Geometry check sheet. Reference: the model listing, model coordinates, mm. A direction names the side the tool comes from. Round coordinates to 2 decimals unless told otherwise and drop trailing zeros. Write each loop counter-clockwise with the first axis right and the second up, starting at its lowest first coordinate (ties: lowest second). Pieces come first, ordered by that corner, then holes.
Item 1: Cross-section at A-A (z = 1.75). State how many separate pieces and enclosed holes the cut face has, then the cut area to 3 significant figures.
Item 2: Cross-section at B-B (y = -4.5). Enter the section's corners in (x, z).
Item 3: Draft check along X on faces 1 (the face through (5.3, 0, 1)), 2 (the face through (0, -1.25, -1)), 3 (the face through (-10, 0, 4)). Enter one of: pulls with the +X half, pulls with the -X half, needs draft (parallel to the pull), parting line crosses it, or undercut.
Item 4: Depth check by flat-ended pin: P1, Ø0.6, axis at x = 5.5, z = 2, coming from the +Y side; P2, Ø0.6, axis at x = 0.5, z = -1.5, coming from the -Y side; P3, Ø0.6, axis at y = -2, z = 1.5, coming from the -X side. Enter the tip coordinate at first touch or a pass-through.
Item 5: Scan lines: probe 1 along Z at (x, y) = (-3.5, 2.25); probe 2 along X at (y, z) = (-2, 2.5); probe 3 along X at (y, z) = (-1.75, 1.5). Record each from-to range of solid material in increasing order.
Item 6: Cross-section at C-C (x = 9). Enter the section's corners in (y, z).
Item 7: Access from +Z, -Z, +X, -X, +Y, -Y to the whole of each face (thin tool, end or side, straight path). Record for faces 4 (the face through (0, 1.25, -1)), 5 (the face through (0, -2, 0)), 6 (the face through (-0.1, -2.1, 2.6)), 7 (the face through (0, -6.5, 4)), 8 (the face through (-5.3, 0, 1)).
from build123d import *

# Parameters (mm, degrees)
F1_DEPTH = 2.6
F2_W     = 10.6
F2_H     = 2.5
F3_DEPTH = 2
F5_DEPTH = 0.6
F7_DEPTH = 2
F9_DEPTH = 2
F9_TAPER = 7


# Not quite as in the source:
# - a feature names something its author has since deleted; it is built from what else it names


with BuildPart() as f1:
    # F0 (on Top) → F1 (new body)
    with BuildSketch(Plane.XY):
        Polygon((6, 2.5), (-6, 2.5), (-6, 1.25), (-5.3, 1.25), (-5.3, -1.25), (-6, -1.25), (-6, -2.5), (6, -2.5), (6, -1.25), (5.3, -1.25), (5.3, 1.25), (6, 1.25), align=None)
    extrude(amount=F1_DEPTH)

    # F2 (on face) → F3 (join)
    with BuildSketch(Plane(origin=(0, 0, 0), x_dir=(1, 0, 0), z_dir=(0, 0, -1))):
        Rectangle(F2_W, F2_H)
    extrude(amount=F3_DEPTH)

    # F4 (on face) → F5 (join)
    with BuildSketch(Plane.XY.offset(2.6)):
        Polygon((5.375, 1.875), (-5.375, 1.875), (-5.375, 1.25), (-5.3, 1.25), (-5.3, -1.25), (-5.375, -1.25), (-5.375, -1.875), (5.375, -1.875), (5.375, -1.25), (5.3, -1.25), (5.3, 1.25), (5.375, 1.25), align=None)
    extrude(amount=F5_DEPTH)

    # F6 (on face) → F7 (join)
    with BuildSketch(Plane.XY.offset(3.2)):
        with BuildLine():
            Line((8.75, 6.5), (-8.75, 6.5))
            ThreePointArc((-8.75, 6.5), (-9.6338834765, 6.1338834765), (-10, 5.25))
            Line((-10, 5.25), (-10, -5.25))
            ThreePointArc((-10, -5.25), (-9.6338834765, -6.1338834765), (-8.75, -6.5))
            Line((-8.75, -6.5), (8.75, -6.5))
            ThreePointArc((8.75, -6.5), (9.6338834765, -6.1338834765), (10, -5.25))
            Line((10, -5.25), (10, 5.25))
            ThreePointArc((10, 5.25), (9.6338834765, 6.1338834765), (8.75, 6.5))
        make_face()
    extrude(amount=F7_DEPTH)

    # F8 (on face) → F9 (join)
    with BuildSketch(Plane(origin=(0, 0, 3.2), x_dir=(1, 0, 0), z_dir=(0, 0, -1))):
        with BuildLine():
            Line((7.25, 4.25), (-7.25, 4.25))
            ThreePointArc((-7.25, 4.25), (-7.6035533906, 4.1035533906), (-7.75, 3.75))
            Line((-7.75, 3.75), (-7.75, -3.75))
            ThreePointArc((-7.75, -3.75), (-7.6035533906, -4.1035533906), (-7.25, -4.25))
            Line((-7.25, -4.25), (7.25, -4.25))
            ThreePointArc((7.25, -4.25), (7.6035533906, -4.1035533906), (7.75, -3.75))
            Line((7.75, -3.75), (7.75, 3.75))
            ThreePointArc((7.75, 3.75), (7.6035533906, 4.1035533906), (7.25, 4.25))
        make_face()
        with BuildLine():
            ThreePointArc((-6.75, 3), (-6.6035533906, 3.3535533906), (-6.25, 3.5))
            Line((-6.25, 3.5), (6.25, 3.5))
            ThreePointArc((6.25, 3.5), (6.6035533906, 3.3535533906), (6.75, 3))
            Line((6.75, 3), (6.75, -3))
            ThreePointArc((6.75, -3), (6.6035533906, -3.3535533906), (6.25, -3.5))
            Line((6.25, -3.5), (-6.25, -3.5))
            ThreePointArc((-6.25, -3.5), (-6.6035533906, -3.3535533906), (-6.75, -3))
            Line((-6.75, -3), (-6.75, 3))
        make_face(mode=Mode.SUBTRACT)
    extrude(amount=F9_DEPTH, taper=F9_TAPER)


solid = f1.part
Resolved:
1. separate pieces: 2
1. enclosed holes: 1
1. area: 78.2 mm2
2. outline: (-10, 3.2) - (10, 3.2) - (10, 5.2) - (-10, 5.2) - close
3. face 1: undercut
3. face 2: needs draft
3. face 3: pulls with the -X half
4. P1: stops at y = 4.14
4. P2: stops at y = -1.25
4. P3: stops at x = -7.58
5. probe 1: z = 0 to 2.6, 3.2 to 5.2
5. probe 2: x = -7.66 to -6.84, -6 to 6, 6.84 to 7.66
5. probe 3: x = -7.54 to -6.96, -6 to 6, 6.96 to 7.54
6. outline: (-6.47, 3.2) - (6.47, 3.2) - (6.47, 5.2) - (-6.47, 5.2) - close
7. face 4: -Z, +X, -X, +Y
7. face 5: -Z, +X, -X, -Y
7. face 6: none
7. face 7: +Z, -Z, +X, -X, -Y
7. face 8: -Z
